from build123d import *

# Parameters (mm, degrees)
SKETCH1_R           = 45
SKETCH1_R_2         = 3.75
BOSS_EXTRUDE1_DEPTH = 6.75
SKETCH3_R           = 6.5
SKETCH2_R           = 20
SKETCH5_R           = 5.5
BOSS_EXTRUDE2_DEPTH = 3
SKETCH6_R           = 4
CUT_EXTRUDE2_DEPTH  = 76.975324942
SKETCH8_R           = 6
CUT_EXTRUDE3_DEPTH  = 2


with BuildPart() as part:
    # Sketch1 → Boss-Extrude1 (new, symmetric)
    with BuildSketch(Plane.XY):
        Circle(SKETCH1_R)
        with Locations((0, 37.5)):
            Circle(SKETCH1_R_2, mode=Mode.SUBTRACT)
        with Locations((11.588137289, 35.664619361)):
            Circle(SKETCH1_R_2, mode=Mode.SUBTRACT)
        with Locations((22.041946961, 30.338137289)):
            Circle(SKETCH1_R_2, mode=Mode.SUBTRACT)
        with Locations((30.338137289, 22.041946961)):
            Circle(SKETCH1_R_2, mode=Mode.SUBTRACT)
        with Locations((35.664619361, 11.588137289)):
            Circle(SKETCH1_R_2, mode=Mode.SUBTRACT)
        with Locations((37.5, 0)):
            Circle(SKETCH1_R_2, mode=Mode.SUBTRACT)
        with Locations((35.664619361, -11.588137289)):
            Circle(SKETCH1_R_2, mode=Mode.SUBTRACT)
        with Locations((30.338137289, -22.041946961)):
            Circle(SKETCH1_R_2, mode=Mode.SUBTRACT)
        with Locations((22.041946961, -30.338137289)):
            Circle(SKETCH1_R_2, mode=Mode.SUBTRACT)
        with Locations((11.588137289, -35.664619361)):
            Circle(SKETCH1_R_2, mode=Mode.SUBTRACT)
        with Locations((0, -37.5)):
            Circle(SKETCH1_R_2, mode=Mode.SUBTRACT)
        with Locations((-11.588137289, -35.664619361)):
            Circle(SKETCH1_R_2, mode=Mode.SUBTRACT)
        with Locations((-22.041946961, -30.338137289)):
            Circle(SKETCH1_R_2, mode=Mode.SUBTRACT)
        with Locations((-30.338137289, -22.041946961)):
            Circle(SKETCH1_R_2, mode=Mode.SUBTRACT)
        with Locations((-35.664619361, -11.588137289)):
            Circle(SKETCH1_R_2, mode=Mode.SUBTRACT)
        with Locations((-37.5, 0)):
            Circle(SKETCH1_R_2, mode=Mode.SUBTRACT)
        with Locations((-35.664619361, 11.588137289)):
            Circle(SKETCH1_R_2, mode=Mode.SUBTRACT)
        with Locations((-30.338137289, 22.041946961)):
            Circle(SKETCH1_R_2, mode=Mode.SUBTRACT)
        with Locations((-22.041946961, 30.338137289)):
            Circle(SKETCH1_R_2, mode=Mode.SUBTRACT)
        with Locations((-11.588137289, 35.664619361)):
            Circle(SKETCH1_R_2, mode=Mode.SUBTRACT)
    extrude(amount=BOSS_EXTRUDE1_DEPTH, both=True)

    # Sketch3 → Loft1 section 0
    with BuildSketch(Plane.XY.offset(31.75)):
        Circle(SKETCH3_R)
    # Sketch2 → Loft1 section 1
    with BuildSketch(Plane.XY.offset(6.75)):
        Circle(SKETCH2_R)
    loft()

    # Sketch5 → Boss-Extrude2 (add)
    with BuildSketch(Plane.XY.offset(31.75)):
        Circle(SKETCH5_R)
    extrude(amount=BOSS_EXTRUDE2_DEPTH)

    # Sketch6 → Cut-Extrude2 (cut, through all)
    with BuildSketch(Plane.XY.offset(34.75)):
        Circle(SKETCH6_R)
    extrude(amount=-CUT_EXTRUDE2_DEPTH, mode=Mode.SUBTRACT)

    # Sketch8 → Cut-Extrude3 (cut)
    with BuildSketch(Plane(origin=(0, 0, -6.75), x_dir=(-1, 0, 0), z_dir=(0, 0, -1))):
        Circle(SKETCH8_R)
    extrude(amount=-CUT_EXTRUDE3_DEPTH, mode=Mode.SUBTRACT)


solid = part.part
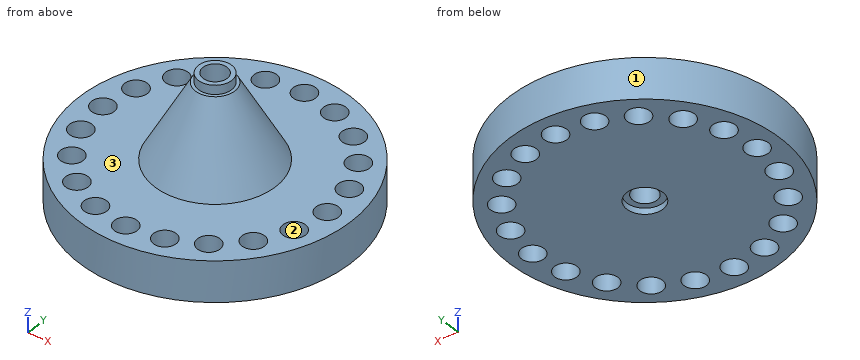
The listing builds one solid part. Answer for the finished solid, in the listing's coordinates (mm). Face numbers are marked on the shaded views. Coordinates: 2 decimals unless noted, no trailing zeros. Loops run counter-clockwise (first coordinate to the right, second up) from the corner with the lowest first, then second, coordinate; pieces in that order, holes last.
1) Find section B-B on y = -37.5. Write down the section's boundary in (x, z).
2) Find section A-A on x = 0. Write down the section's boundary in (y, z), then the cut area to 3 significant figures.
3) Find section D-D on x = -38. Write down the section's boundary in (y, z), then the cut area to 3 significant figures.
4) Find section C-C on z = 3.5. Give the number of separate pieces and of enclosed holes in the cut face, then the cut area to 3 significant figures.
5) Flat-ended cylindrical pins translate along their axes: pin 1 Ø3.5 at (x, y) = (3, 2) entering from -Z; pin 2 Ø3 at (x, y) = (-2.5, 27) entering from +Z; pin 3 Ø12 at (x, z) = (32, 4) entering from +Y. Find the tip coordinate at first contact, or state that the pin passes through.
6) Determine the mould class of the marked faces 1, 2 and 3 for opening direction Y: pulls with the +Y half, pulls with the -Y half, needs draft (parallel to the pull), parting line crosses it, or undercut.
7) Find the intervals of material crossed by L1, parallel to Y at x = 9, z = -0.5; L2, parallel to Y at x = 38, z = -4; L3, parallel to X at y = 15, z = 4.5, in increasing order.
Values:
1. outline: (-24.87, -6.75) - (-14.86, -6.75) - (-14.86, 6.75) - (-24.87, 6.75) - close; (-8.32, -6.75) - (-3.75, -6.75) - (-3.75, 6.75) - (-8.32, 6.75) - close; (3.75, -6.75) - (8.32, -6.75) - (8.32, 6.75) - (3.75, 6.75) - close; (14.86, -6.75) - (24.87, -6.75) - (24.87, 6.75) - (14.86, 6.75) - close
2. outline: (-45, -6.75) - (-41.25, -6.75) - (-41.25, 6.75) - (-45, 6.75) - close; (-33.75, -6.75) - (-6, -6.75) - (-6, -4.75) - (-4, -4.75) - (-4, 34.75) - (-5.5, 34.75) - (-5.5, 31.75) - (-6.5, 31.75) - (-20, 6.75) - (-33.75, 6.75) - close; (4, -4.75) - (6, -4.75) - (6, -6.75) - (33.75, -6.75) - (33.75, 6.75) - (20, 6.75) - (6.5, 31.75) - (5.5, 31.75) - (5.5, 34.75) - (4, 34.75) - close; (41.25, -6.75) - (45, -6.75) - (45, 6.75) - (41.25, 6.75) - close
2. area: 1,370 mm2
3. outline: (-24.1, -6.75) - (-14.52, -6.75) - (-14.52, 6.75) - (-24.1, 6.75) - close; (-8.65, -6.75) - (-3.72, -6.75) - (-3.72, 6.75) - (-8.65, 6.75) - close; (3.72, -6.75) - (8.65, -6.75) - (8.65, 6.75) - (3.72, 6.75) - close; (14.52, -6.75) - (24.1, -6.75) - (24.1, 6.75) - (14.52, 6.75) - close
3. area: 392 mm2
4. separate pieces: 1
4. enclosed holes: 21
4. area: 5,430 mm2
5. pin 1: stops at z = -4.75
5. pin 2: stops at z = 6.75
5. pin 3: stops at y = 36.73
6. face 1: parting line crosses it
6. face 2: undercut
6. face 3: needs draft
7. L1: y = -44.09 to -38.38, -32.95 to 32.95, 38.38 to 44.09
7. L2: y = -24.1 to -14.52, -8.65 to -3.72, 3.72 to 8.65, 14.52 to 24.1
7. L3: x = -42.43 to -37.22, -34.11 to 34.11, 37.22 to 42.43
